The model under review builds one solid part; all positions refer to its coordinate system, in mm. A direction names the side the tool comes from. Give positions to 0.01 mm unless a question says otherwise; leave off trailing zeros. Loops run counter-clockwise (first coordinate to the right, second up) from the corner with the lowest first, then second, coordinate; pieces in that order, holes last. Notation, with made-up numbers: M 7.5,0 L 39.5,0 A23 ccw 39.5,21 Z; hole C 87,73 d7. An arc over 180 degrees is marked long. Return JSON: item names as keys, results as strings.
Autodesk Inventor part; units mm, degrees
ref_plane "YZ Plane" through (0, 0, 0) normal (1, 0, 0) x (0, 1, 0)
ref_plane "XZ Plane" through (0, 0, 0) normal (0, 1, 0) x (-1, 0, 0)
ref_plane "XY Plane" through (0, 0, 0) normal (0, 0, 1) x (1, 0, 0)
sketch "Sketch1" plane through (0, 0, 0) normal (0, 1, 0) x (-1, 0, 0)
  line L0 (0, 0) -> (16, 0)
  line L1 (16, 0) -> (16, -20)
  line L2 (16, -20) -> (0, -20)
  line L3 (0, -20) -> (0, 0)
  dimension "d0" = 16
  dimension "d1" = 20
extrude "Extrusion1" add sketch "Sketch1" along normal blind 11.5
sketch "Sketch2" plane through (0, 11.5, 0) normal (0, 1, 0) x (1, 0, 0)
  line L0 (0, 0) -> (0, 20)
  line L1 (0, 20) -> (-16, 20)
  circle A0 centre (-8, 15.5) radius 3
  dimension "d4" = 6
  dimension "d5" = 8
  dimension "d6" = 4.5
extrude "Extrusion2" cut sketch "Sketch2" against normal up to surface (11.5 mm away)
sketch "Sketch3" plane through (0, 11.5, 0) normal (0, 1, 0) x (1, 0, 0)
  line L0 (0, 0) -> (0, 20)
  line L1 (0, 20) -> (-16, 20)
  circle A0 centre (-8, 2.5) radius 1.5
  dimension "d9" = 3
  dimension "d11" = 17.5
  dimension "d12" = 8
extrude "Extrusion3" cut sketch "Sketch3" against normal up to surface (11.5 mm away)
sketch "Sketch4" plane through (0, 0, 0) normal (1, 0, 0) x (0, 0, -1)
  line L0 (20, 0) -> (0, 0)
  line L1 (20, 0) -> (20, 11.5)
  line L2 (0, 0) -> (0, 11.5)
  arc A0 (5.5953, 3.25) -> (5.5953, 4.75) centre (8.5, 4) ccw
  line L3 (5.5953, 4.75) -> (0, 4.75)
  line L4 (5.5953, 3.25) -> (0, 3.25)
  dimension "d15" = 6
  dimension "d16" = 11.5
  dimension "d17" = 4
  dimension "d18" = 1.5
  dimension "d19" = 0.75
extrude "Extrusion4" cut sketch "Sketch4" against normal up to surface (16 mm away)
sketch "Sketch5" plane through (0, 0, 0) normal (1, 0, 0) x (0, 0, -1)
  line L0 (20, 0) -> (0, 0)
  line L1 (20, 0) -> (20, 11.5)
  circle A0 centre (18, 2) radius 0.75
  dimension "d22" = 1.5
  dimension "d24" = 2
  dimension "d25" = 2
extrude "Extrusion5" cut sketch "Sketch5" against normal blind 4.4
sketch "Sketch6" plane through (0, 0, 0) normal (1, 0, 0) x (0, 0, -1)
  line L0 (20, 0) -> (0, 0)
  line L1 (20, 0) -> (20, 11.5)
  circle A0 centre (16.5, 4.8) radius 1.5
  dimension "d28" = 3
  dimension "d29" = 4.8
  dimension "d30" = 3.5
extrude "Extrusion6" cut sketch "Sketch6" against normal blind 3.4
thread "Thread1"
thread "Thread2"
thread "Thread3"
properties part number "E3DV6NozzleBlock" material "Aluminum 6061"
1) Insertion check: pin 1 (1.8 mm diameter, centred on x = -8, z = -2.5, fed in from -Y); pin 2 (1.8 mm diameter, centred on y = 4.8, z = -16.5, fed in from +X). Each pin has a flat end and moves straight along its axis. Give the tip position at first contact, or say it passes through.
From the geometry:
{"pin 1": "through", "pin 2": "x = -3.4"}
2) Wall thickness on L1, parallel to X at y = 3.5, z = -15.5; L2, parallel to Y at x = -10, z = -5.5; L3, parallel to Z at x = -8.5, y = 10.75: over which ranges is each line inside the solid? List them lowest first. Write a range as from..to.
From the geometry:
{"L1": "-16..-11, -5..0", "L2": "0..3.25, 4.75..11.5", "L3": "-20..-18.46, -12.54..-3.91, -1.09..0"}
3) Tool access review of faces 5 (the face through (-1.68, 5.81, -15.39)), 6 (the face through (-10, 4.75, -3)), 7 (the face through (-9.2, 8.2, -1.6)): name each direction out of +Z, -Z, +X, -X, +Y, -Y from which nothing blocks a thin tool from reaching the whole face with its end or side.
From the geometry:
{"face 5": "+X", "face 6": "+Z, +X, -X", "face 7": "+Y, -Y"}
4) Consider section C-C on x = -8. Write out the cut boundary in (y, z), then the cut area to 3 significant figures.
From the geometry:
{"outline": "M 0,-20 L 11.5,-20 L 11.5,-18.5 L 0,-18.5 Z; M 0,-12.5 L 11.5,-12.5 L 11.5,-4 L 4.75,-4 L 4.75,-5.6 A3 cw long 3.25,-5.6 L 3.25,-4 L 0,-4 Z; M 0,-1 L 3.25,-1 L 3.25,0 L 0,0 Z; M 4.75,-1 L 11.5,-1 L 11.5,0 L 4.75,0 Z", "area": "94.4 mm²"}
5) Consider section A-A on z = -8.5. Write out the cut boundary in (x, y), then the cut area to 3 significant figures.
From the geometry:
{"outline": "M -16,0 L 0,0 L 0,1 L -16,1 Z; M -16,7 L 0,7 L 0,11.5 L -16,11.5 Z", "area": "88.0 mm²"}
6) Consider section B-B on y = 1.5. Write out the cut boundary in (x, z), then the cut area to 3 significant figures.
From the geometry:
{"outline": "M -16,-20 L 0,-20 L 0,-18.56 L -4.4,-18.56 L -4.4,-17.44 L 0,-17.44 L 0,-10.16 L -16,-10.16 Z; M -16,-6.84 L 0,-6.84 L 0,0 L -16,0 Z; hole C -8,-15.5 d6; hole C -8,-2.5 d3", "area": "227 mm²"}
7) The part is to be moulded in two halves that separate along Y. For faces 1 (the face through (-8, 6, -20)), 2 (the face through (-3.4, 5, -16)), 3 (the face through (-4.4, 2, -18)), 4 (the face through (-8, 11.5, -10)), say which applies: released by +Y, released by -Y, zero draft, split by the parting line, or undercut.
From the geometry:
{"face 1": "zero draft", "face 2": "undercut", "face 3": "undercut", "face 4": "released by +Y"}
8) Consider section D-D on x = -6. Write out the cut boundary in (y, z).
From the geometry:
{"outline": "M 0,-20 L 11.5,-20 L 11.5,-17.74 L 0,-17.74 Z; M 0,-13.26 L 11.5,-13.26 L 11.5,0 L 4.75,0 L 4.75,-5.6 A3 cw long 3.25,-5.6 L 3.25,0 L 0,0 Z"}
